Source: three-view drawing plus pictorial views. Frame: mm from the lowest corner of the part. Coordinates: 2 decimals unless noted, no trailing zeros. Write each loop counter-clockwise with the first axis right and the second up, starting at its lowest first coordinate (ties: lowest second). Pieces come first, ordered by that corner, then holes. Notation, with made-up numbers: (56, 22) - (104, 22) arc R17 ccw to (104, 45) - close; hole circle Ø1 at (4.5, 43.25). An arc over 180 degrees is marked (long way). Put each result on its own line as item: value. Start each with the question number.
1. Pin query (flat end, axial travel): pin 1 (0.9 mm diameter, centred on y = 1, z = 3, fed in from -X); pin 2 (3 mm diameter, centred on x = 49, z = 3.5, fed in from -Y); pin 3 (1.5 mm diameter, centred on x = 75, y = 2, fed in from -Z). Return the tip coordinate at first contact, or that it passes through.
2. Pull-direction query (Z, two-part tool) for the marked faces 1 and 2; classes: released by +Z, released by -Z, zero draft, split by the parting line, or undercut.
3. Line query: line 1 (Z direction, x = 49, y = 8); line 2 (Y direction, x = 14.5, z = 0.8); line 3 (X direction, y = 21.5, z = 0.6). Output: solid intervals per line, ascending.
4. Cut plane A-A, the plane x = 49. Return loops of the section in (y, z).
5. Cut plane D-D, the plane x = 27.5. Return loops of the section in (y, z), and give its area (3 significant figures).
6. Cut plane B-B, the plane z = 3. Return loops of the section in (x, y), and give its area (3 significant figures).
7. Cut plane C-C, the plane y = 34. Return loops of the section in (x, z).
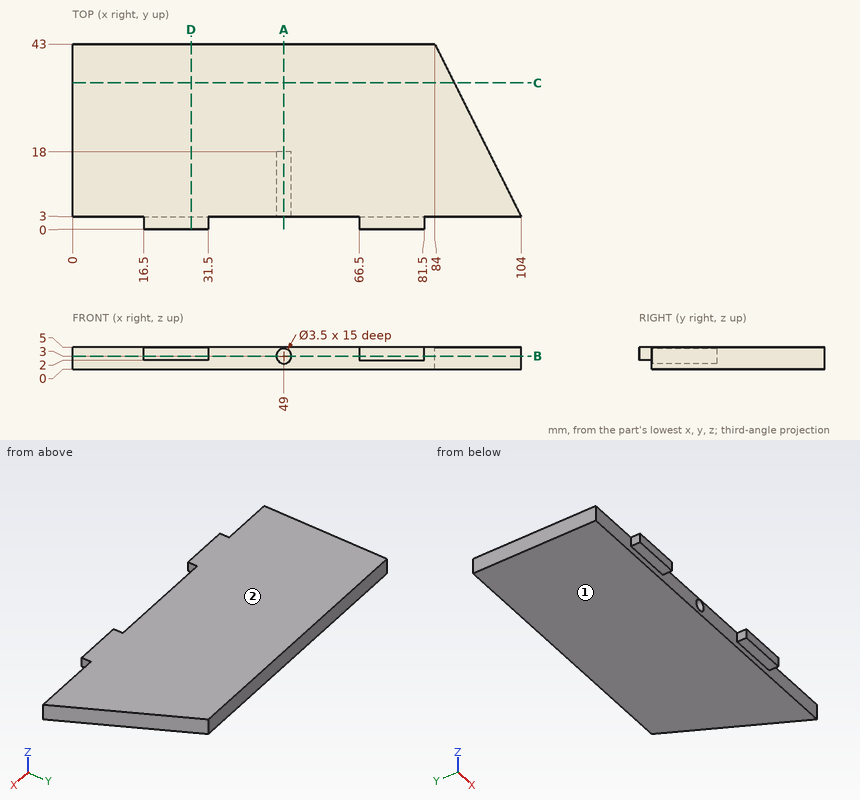
Report:
1. pin 1: stops at x = 16.5
1. pin 2: stops at y = 3
1. pin 3: stops at z = 2
2. face 1: released by -Z
2. face 2: released by +Z
3. line 1: z = 0 to 1.25, 4.75 to 5
3. line 2: y = 3 to 43
3. line 3: x = 0 to 94.75
4. outline: (3, 0) - (43, 0) - (43, 5) - (3, 5) - (3, 4.75) - (18, 4.75) - (18, 1.25) - (3, 1.25) - close
5. outline: (0, 2) - (3, 2) - (3, 0) - (43, 0) - (43, 5) - (0, 5) - close
5. area: 209 mm^2
6. outline: (0, 3) - (16.5, 3) - (16.5, 0) - (31.5, 0) - (31.5, 3) - (47.25, 3) - (47.25, 18) - (50.75, 18) - (50.75, 3) - (66.5, 3) - (66.5, 0) - (81.5, 0) - (81.5, 3) - (104, 3) - (84, 43) - (0, 43) - close
6. area: 3,800 mm^2
7. outline: (0, 0) - (88.5, 0) - (88.5, 5) - (0, 5) - close
